```python
from build123d import *

# Parameters (mm, degrees)
SKETCH1_R           = 8.345
BOSS_EXTRUDE1_DEPTH = 25
CUT_EXTRUDE3_START  = -11
CUT_EXTRUDE3_DEPTH  = 22
SKETCH3_R           = 10
BOSS_EXTRUDE2_DEPTH = 40


# Read off the part's stored shape, not the designer's step: Cut-Extrude3
with BuildPart() as part:
    # Sketch1 → Boss-Extrude1 (new body)
    with BuildSketch(Plane(origin=(0, 0, 0), x_dir=(0, 0, -1), z_dir=(1, 0, 0))):
        with BuildLine():
            Line((-15.282961101, -11), (-55.282961101, -11))
            Line((-55.282961101, -11), (-55.282961101, 11))
            Line((-55.282961101, 11), (-15.282961101, 11))
            ThreePointArc((-15.282961101, 11), (18.83, 0), (-15.282961101, -11))
        make_face()
        Circle(SKETCH1_R, mode=Mode.SUBTRACT)
    extrude(amount=BOSS_EXTRUDE1_DEPTH)

    # Cut-Extrude3 outline → Cut-Extrude3 (cut)
    with BuildSketch(Plane(origin=(0, 0, 0), x_dir=(1, 0, 0), z_dir=(0, 1, 0)).offset(CUT_EXTRUDE3_START)):
        with BuildLine():
            Line((25, -55.282961101), (25, -15.282961101))
            Line((25, -15.282961101), (24.5, -15.282961101))
            ThreePointArc((24.5, -15.282961101), (23.792893218, -15.575854319), (23.5, -16.282961101))
            Line((23.5, -16.282961101), (23.5, -55.282961101))
            Line((23.5, -55.282961101), (25, -55.282961101))
        make_face()
        with BuildLine():
            Line((0, -55.282961101), (1.5, -55.282961101))
            Line((1.5, -55.282961101), (1.5, -16.282961101))
            ThreePointArc((1.5, -16.282961101), (1.207106782, -15.575854319), (0.5, -15.282961101))
            Line((0.5, -15.282961101), (0, -15.282961101))
            Line((0, -15.282961101), (0, -55.282961101))
        make_face()
    extrude(amount=CUT_EXTRUDE3_DEPTH, mode=Mode.SUBTRACT)

    # Sketch3 → Boss-Extrude2 (add)
    with BuildSketch(Plane.XY.offset(55.282961101)):
        with Locations((12.5, 0)):
            Circle(SKETCH3_R)
    extrude(amount=BOSS_EXTRUDE2_DEPTH)


solid = part.part
```
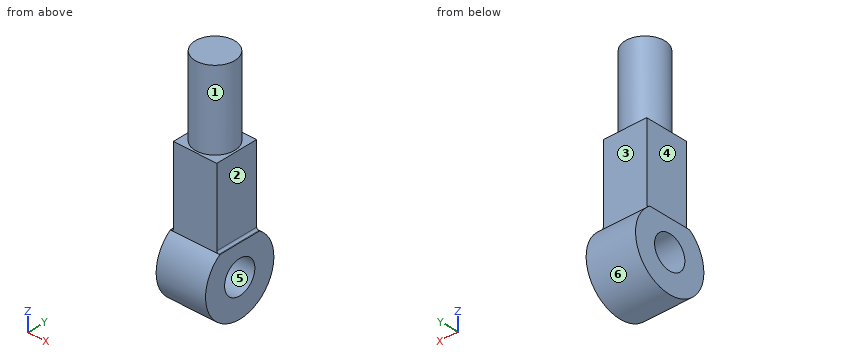
Here's how the part is built. I have some questions about the finished solid (model axes, mm). Face numbers are marked on the shaded views. A direction names the side the tool comes from. Give positions to 0.01 mm unless a question says otherwise; leave off trailing zeros. Loops run counter-clockwise (first coordinate to the right, second up) from the corner with the lowest first, then second, coordinate; pieces in that order, holes last. Notation, with made-up numbers: M 82,41 L 117,41 A12 cw 117,47 Z; hole C 82.5,45 d1. An arc over 180 degrees is marked long. Return JSON: item names as keys, results as strings.
Item 1: On a 3-axis mill with a long thin cutter (end or side, diameter ignored), from which of +Z, -Z, +X, -X, +Y, -Y can I reach the whole of each face in a straight line? I mean the marked faces 1, 2 and 3. Say none if no direction works.
A:
{"face 1": "+Z", "face 2": "+Z, +X, +Y, -Y", "face 3": "+Z, +X, -X, +Y"}
Item 2: Thinking about a two-plate mould opening in Y: for the marked faces 4, 5 and 6, which applies, released by +Y, released by -Y, zero draft, split by the parting line, or undercut?
A:
{"face 4": "zero draft", "face 5": "undercut", "face 6": "split by the parting line"}
Item 3: Imagine slicing it at C-C on x = 12.5. List the corners of the cut face in (y, z) for me (3 decimals), then the cut area to 3 significant figures.
A:
{"outline": "M -11,15.283 A18.83 ccw long 11,15.283 L 11,55.283 L 10,55.283 L 10,95.283 L -10,95.283 L -10,55.283 L -11,55.283 Z; hole C 0,0 d16.69", "area": "2,520 mm^2"}
Item 4: I'm going to push flat-ended pins straight in: pin 1 Ø11 at (y, z) = (1, 29.5) entering from +X; pin 2 Ø6.5 at (y, z) = (1, 42.5) entering from -X; pin 3 Ø0.6 at (x, y) = (0.5, 4) entering from +Z; pin 4 Ø10 at (y, z) = (0, 0) entering from +X. Where does each tip first touch, or does it pass through?
A:
{"pin 1": "stops at x = 23.5", "pin 2": "stops at x = 1.5", "pin 3": "stops at z = 15.33", "pin 4": "passes through"}
Item 5: Imagine slicing it at A-A on z = 0. List the corners of the cut face in (x, y) for me (3 decimals).
A:
{"outline": "M 0,-18.83 L 25,-18.83 L 25,-8.345 L 0,-8.345 Z; M 0,8.345 L 25,8.345 L 25,18.83 L 0,18.83 Z"}
Item 6: Imagine slicing it at D-D on z = 68. List the corners of the cut face in (x, y) for me, then the cut area to 3 significant figures.
A:
{"outline": "C 12.5,0 d20", "area": "314 mm^2"}
Item 7: Imagine slicing it at B-B on y = 0. List the corners of the cut face in (x, z) for me (3 decimals), then the cut area to 3 significant figures.
A:
{"outline": "M 0,-18.83 L 25,-18.83 L 25,-8.345 L 0,-8.345 Z; M 0,8.345 L 25,8.345 L 25,15.283 L 24.5,15.283 A1 cw 23.5,16.283 L 23.5,55.283 L 22.5,55.283 L 22.5,95.283 L 2.5,95.283 L 2.5,55.283 L 1.5,55.283 L 1.5,16.283 A1 cw 0.5,15.283 L 0,15.283 Z", "area": "2,120 mm^2"}
Item 8: Please list where these lines run through material, in increasing order: line 1 (Y direction, x = 18.75, z = 0) (3 decimals); line 2 (X direction, y = -10, z = 29.5); line 3 (Y direction, x = 22.5, z = 44.5).
A:
{"line 1": "y = -18.83 to -8.345, 8.345 to 18.83", "line 2": "x = 1.5 to 23.5", "line 3": "y = -11 to 11"}
